Part print with two shaded views. Sizes in mm from the minimum x, y, z corner. A direction names the side the tool comes from. Round coordinates to 2 decimals unless told otherwise and drop trailing zeros. Write each loop counter-clockwise with the first axis right and the second up, starting at its lowest first coordinate (ties: lowest second). Pieces come first, ordered by that corner, then holes. Notation, with made-up numbers: (18, 89.5) - (47, 89.5) arc R25 cw to (47, 108.5) - close; hole circle Ø11 at (31.5, 58.25). An arc over 180 degrees is marked (long way). Use one line per item in the form item = value. Start each with the question number.
Item 1: Drill centre lines: L1, parallel to X at y = 3.5, z = 12.25 (1 decimal); L2, parallel to Z at x = 15, y = 8; L3, parallel to X at y = 2.5, z = 11.25 (1 decimal). Where is each one in solid material? Low to high.
Item 2: Band-saw the part on A-A, the plane x = 15. List the corners of the cut face in (y, z) (1 decimal), and give its area (3 significant figures).
Item 3: Pin check, flat tips, straight feed: pin 1 (13 mm diameter, centred on x = 142.97, z = 15, fed in from -Y); pin 2 (7 mm diameter, centred on x = 10, z = 8, fed in from +Y) (1 decimal); pin 3 (4 mm diameter, centred on y = 44, z = 7, fed in from -X) (1 decimal); pin 4 (6 mm diameter, centred on x = 15, z = 15, fed in from -Y). Stop position of each tip, or through.
Item 4: Band-saw the part on C-C, the plane y = 10. List the corners of the cut face in (x, z) (1 decimal).
Item 5: Pull direction Z, two halves, no side cores. Call the marked faces 1, 2 and 3: +Z half, -Z half, draft (parallel to the pull), parting line (faces both ways), or undercut.
Item 6: Band-saw the part on B-B, the plane z = 15. List the corners of the cut face in (x, y) (1 decimal).
Item 7: Band-saw the part on D-D, the plane y = 23. List the corners of the cut face in (x, z).
Item 8: Tool access for the marked faces 4 and 5: list every direction of +Z, -Z, +X, -X, +Y, -Y with a clear straight run to the whole face (end or side of a thin tool).
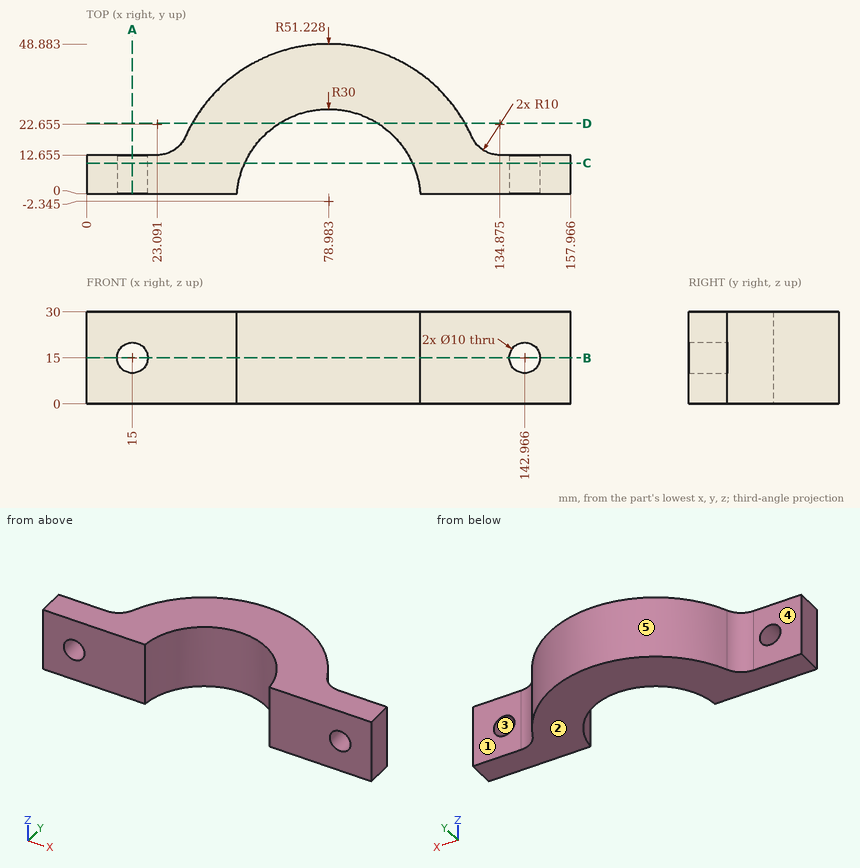
Determined:
q1.L1 = 0 to 10.8, 19.2 to 49.6, 108.4 to 138.8, 147.1 to 158
q1.L2 = 0 to 10, 20 to 30
q1.L3 = 0 to 11.7, 18.3 to 49.4, 108.6 to 139.7, 146.3 to 158
q2.outline = (0, 0) - (12.7, 0) - (12.7, 10) - (0, 10) - close; (0, 20) - (12.7, 20) - (12.7, 30) - (0, 30) - close
q2.area = 253 mm²
q3.pin_1 = 0
q3.pin_2 = 12.7
q3.pin_3 = 53.3
q3.pin_4 = through
q4.outline = (0, 0) - (51.6, 0) - (51.6, 30) - (0, 30) - close; (106.3, 0) - (158, 0) - (158, 30) - (106.3, 30) - close; hole circle Ø10 at (15, 15); hole circle Ø10 at (143, 15)
q5.face_1 = draft
q5.face_2 = -Z half
q5.face_3 = undercut
q6.outline = (0, 0) - (10, 0) - (10, 12.7) - (0, 12.7) - close; (20, 0) - (49.1, 0) arc R30 cw to (108.9, 0) - (138, 0) - (138, 12.7) - (134.9, 12.7) arc R10 cw to (125.7, 18.6) arc R51.2 ccw to (32.2, 18.6) arc R10 cw to (23.1, 12.7) - (20, 12.7) - close; (148, 0) - (158, 0) - (158, 12.7) - (148, 12.7) - close
q7.outline = (34.46, 0) - (62.93, 0) - (62.93, 30) - (34.46, 30) - close; (95.03, 0) - (123.5, 0) - (123.5, 30) - (95.03, 30) - close
q8.face_4 = +Z, -Z, -X, +Y
q8.face_5 = +Z, -Z, +Y
